Here's how the part is built. I have some questions about the finished solid (model axes, mm). A direction names the side the tool comes from. Round coordinates to 2 decimals unless told otherwise and drop trailing zeros. Loops run counter-clockwise (first coordinate to the right, second up) from the corner with the lowest first, then second, coordinate; pieces in that order, holes last. Notation, with made-up numbers: M -26.5,-28.75 L -20.5,-28.75 A19 ccw -20.5,5.25 Z; hole C 30.25,45.5 d4. An arc over 180 degrees is marked long. Answer as a JSON object with one key per item and string values.
from build123d import *

# Parameters (mm, degrees)
SKETCH015_W     = 55.4
SKETCH015_H     = 28.6
PAD011_DEPTH    = 2
SKETCH016_W     = 55.4
SKETCH016_H     = 28.6
SKETCH016_W_2   = 51.4
SKETCH016_H_2   = 24.6
PAD012_DEPTH    = 2.75
SKETCH019_W     = 10
SKETCH019_H     = 15
POCKET006_DEPTH = 2


with BuildPart() as part:
    # Sketch015 → Pad011 (new body)
    with BuildSketch(Plane.XY):
        Rectangle(SKETCH015_W, SKETCH015_H)
    extrude(amount=PAD011_DEPTH)

    # Sketch016 (on Face6 of Pad011) → Pad012 (join)
    with BuildSketch(Plane.XY.offset(2)):
        Rectangle(SKETCH016_W, SKETCH016_H)
        Rectangle(SKETCH016_W_2, SKETCH016_H_2, mode=Mode.SUBTRACT)
    extrude(amount=PAD012_DEPTH)

    # Sketch019 (on Face15 of Pad012) → Pocket006 (cut)
    with BuildSketch(Plane.XY.offset(2)):
        with Locations((-20.7, 0)):
            Rectangle(SKETCH019_W, SKETCH019_H)
        with Locations((20.7, 0)):
            Rectangle(SKETCH019_W, SKETCH019_H)
    extrude(amount=-POCKET006_DEPTH, mode=Mode.SUBTRACT)


solid = part.part
Item 1: If we mould it in two halves opening along Y, with no side actions, what happens to faces 1 (the face through (-21, -7.5, 1)), 2 (the face through (27.7, 0, 2)), 3 (the face through (0, 14.3, 2))? For each: pulls with the +Y half, pulls with the -Y half, needs draft (parallel to the pull), parting line crosses it, or undercut.
Resolved:
{"face 1": "undercut", "face 2": "needs draft", "face 3": "pulls with the +Y half"}
Item 2: On a 3-axis mill with a long thin cutter (end or side, diameter ignored), from which of +Z, -Z, +X, -X, +Y, -Y can I reach the whole of each face in a straight line? I mean faces 4 (the face through (25.7, 0, 3)), 5 (the face through (0, 0, 0)), 6 (the face through (-15.7, 0, 1)). Say none if no direction works.
Resolved:
{"face 4": "+Z", "face 5": "-Z, +X, -X, +Y, -Y", "face 6": "+Z, -Z"}
Item 3: Please list where these lines run through material, in increasing order: probe 1 along X at (y, z) = (-6.75, 1.75); probe 2 along Y at (x, z) = (-24, 1.5); probe 3 along Y at (x, z) = (-16, 3.8). Write a range as from..to.
Resolved:
{"probe 1": "-27.7..-25.7, -15.7..15.7, 25.7..27.7", "probe 2": "-14.3..-7.5, 7.5..14.3", "probe 3": "-14.3..-12.3, 12.3..14.3"}
Item 4: I want a section at B-B, the plane z = 3.6. Please give me the cut outline in (x, y).
Resolved:
{"outline": "M -27.7,-14.3 L 27.7,-14.3 L 27.7,14.3 L -27.7,14.3 Z; hole M -25.7,-12.3 L 25.7,-12.3 L 25.7,12.3 L -25.7,12.3 Z"}
Item 5: I want a section at A-A, the plane y = 5.75. Please give me the cut outline in (x, z).
Resolved:
{"outline": "M -27.7,0 L -25.7,0 L -25.7,4.75 L -27.7,4.75 Z; M -15.7,0 L 15.7,0 L 15.7,2 L -15.7,2 Z; M 25.7,0 L 27.7,0 L 27.7,4.75 L 25.7,4.75 Z"}
Item 6: I want a section at D-D, the plane z = 0.7. Please give me the cut outline in (x, y).
Resolved:
{"outline": "M -27.7,-14.3 L 27.7,-14.3 L 27.7,14.3 L -27.7,14.3 Z; hole M -25.7,-7.5 L -15.7,-7.5 L -15.7,7.5 L -25.7,7.5 Z; hole M 15.7,-7.5 L 25.7,-7.5 L 25.7,7.5 L 15.7,7.5 Z"}
Item 7: I want a section at C-C, the plane x = -16.5. Please give me the cut outline in (y, z), then the cut area to 3 significant figures.
Resolved:
{"outline": "M -14.3,0 L -7.5,0 L -7.5,2 L -12.3,2 L -12.3,4.75 L -14.3,4.75 Z; M 7.5,0 L 14.3,0 L 14.3,4.75 L 12.3,4.75 L 12.3,2 L 7.5,2 Z", "area": "38.2 mm²"}
Item 8: I'm going to push a flat-ended pin straight in: pin 1 Ø4 at (x, y) = (8.5, 9) entering from +Z. Where does the tip first touch, or does it pass through?
Resolved:
{"pin 1": "z = 2"}
